Work out the finished part from the listing and answer in its coordinate system (mm). Round coordinates to 2 decimals unless told otherwise and drop trailing zeros. Order: outer loops, then holes, each group sorted by start corner. A loop starts at its lowest first (then second) coordinate and runs counter-clockwise, first axis right, second up. Notation, with made-up numbers: (19.5, 61) - (53.5, 61) arc R26 cw to (53.5, 100) - close; hole circle Ø1 at (-36.75, 45.25). An arc over 180 degrees is marked (long way). Use CSV: the item, a comma, the result in double quotes.
from build123d import *

# Parameters (mm, degrees)
SKETCH_2_R          = 38.5
SKETCH_2_R_2        = 6.5
SKETCH_2_R_3        = 1.5
EXTRUDE_1_DEPTH     = 2
CHAMFER_1_SIZE      = 2
CHAMFER_1_SIZE_2    = 1.93137755
SKETCH_3_R          = 1.7
EXTRUDE_2_DEPTH     = 2
FILLET_1_R          = 5
CUT_EXTRUDE_1_DEPTH = 10
FILLET_2_R          = 2
CUT_EXTRUDE_4_DEPTH = 10


with BuildPart() as part:
    # 草图2 → 凸台-拉伸1 (new body)
    with BuildSketch(Plane(origin=(0, 0, 0), x_dir=(1, 0, 0), z_dir=(0, 1, 0))):
        with Locations(Location((0, 0, 0), (0, 0, 270))):
            Circle(SKETCH_2_R)
        with Locations(Location((0, 0, 0), (0, 0, 270))):
            Circle(SKETCH_2_R_2, mode=Mode.SUBTRACT)
        with Locations(Location((9.5, 0, 0), (0, 0, 270))):
            Circle(SKETCH_2_R_3, mode=Mode.SUBTRACT)
        with Locations(Location((-4.75, -8.227241336, 0), (0, 0, 270))):
            Circle(SKETCH_2_R_3, mode=Mode.SUBTRACT)
        with Locations(Location((-4.75, 8.227241336, 0), (0, 0, 270))):
            Circle(SKETCH_2_R_3, mode=Mode.SUBTRACT)
    extrude(amount=EXTRUDE_1_DEPTH)

    # 倒角1
    # the kernel refuses this chamfer: 2, 1.93137755 mm, written as the material it takes off along each edge
    with BuildSketch(Plane(origin=(-4.75, 0, 8.227241336), x_dir=(0, 0, 1), z_dir=(-1, 0, 0))) as chamfer_1_piece_1:
        Polygon((1.5, CHAMFER_1_SIZE), (1.5 + CHAMFER_1_SIZE_2, 0), (1.5, 0), align=None)
    revolve(axis=Axis((-4.75, 0, 8.227241336), (0, 1, 0)), mode=Mode.SUBTRACT)
    with BuildSketch(Plane(origin=(-4.75, 0, -8.227241336), x_dir=(0, 0, 1), z_dir=(-1, 0, 0))) as chamfer_1_piece_2:
        Polygon((1.5, CHAMFER_1_SIZE), (1.5 + CHAMFER_1_SIZE_2, 0), (1.5, 0), align=None)
    revolve(axis=Axis((-4.75, 0, -8.227241336), (0, 1, 0)), mode=Mode.SUBTRACT)
    with BuildSketch(Plane(origin=(9.5, 0, 0), x_dir=(0, 0, 1), z_dir=(-1, 0, 0))) as chamfer_1_piece_3:
        Polygon((1.5, CHAMFER_1_SIZE), (1.5 + CHAMFER_1_SIZE_2, 0), (1.5, 0), align=None)
    revolve(axis=Axis((9.5, 0, 0), (0, 1, 0)), mode=Mode.SUBTRACT)

    # 草图3 → 凸台-拉伸2 (add)
    # profile 1 of 4: a face of its own
    with BuildSketch(Plane(origin=(0, 0, 0), x_dir=(1, 0, 0), z_dir=(0, 1, 0))):
        with BuildLine():
            Line((44.5, 3.5), (38.340579025, 3.5))
            ThreePointArc((38.340579025, 3.5), (38.5, 0), (38.340579025, -3.5))
            Line((38.340579025, -3.5), (44.5, -3.5))
            ThreePointArc((44.5, -3.5), (48, 0), (44.5, 3.5))
        make_face()
        with Locations(Location((44.5, 0, 0), (0, 0, 270))):
            Circle(SKETCH_3_R, mode=Mode.SUBTRACT)
    # profile 2 of 4: a face of its own
    with BuildSketch(Plane(origin=(0, 0, 0), x_dir=(1, 0, 0), z_dir=(0, 1, 0))):
        with BuildLine():
            Line((-3.5, 44.5), (-3.5, 38.340579025))
            ThreePointArc((-3.5, 38.340579025), (0, 38.5), (3.5, 38.340579025))
            Line((3.5, 38.340579025), (3.5, 44.5))
            ThreePointArc((3.5, 44.5), (0, 48), (-3.5, 44.5))
        make_face()
        with Locations(Location((0, 44.5, 0), (0, 0, 270))):
            Circle(SKETCH_3_R, mode=Mode.SUBTRACT)
    # profile 3 of 4: a face of its own
    with BuildSketch(Plane(origin=(0, 0, 0), x_dir=(1, 0, 0), z_dir=(0, 1, 0))):
        with BuildLine():
            Line((3.5, -44.5), (3.5, -38.340579025))
            ThreePointArc((3.5, -38.340579025), (0, -38.5), (-3.5, -38.340579025))
            Line((-3.5, -38.340579025), (-3.5, -44.5))
            ThreePointArc((-3.5, -44.5), (0, -48), (3.5, -44.5))
        make_face()
        with Locations(Location((0, -44.5, 0), (0, 0, 270))):
            Circle(SKETCH_3_R, mode=Mode.SUBTRACT)
    # profile 4 of 4: a face of its own
    with BuildSketch(Plane(origin=(0, 0, 0), x_dir=(1, 0, 0), z_dir=(0, 1, 0))):
        with BuildLine():
            Line((-44.5, -3.5), (-38.340579025, -3.5))
            ThreePointArc((-38.340579025, -3.5), (-38.5, 0), (-38.340579025, 3.5))
            Line((-38.340579025, 3.5), (-44.5, 3.5))
            ThreePointArc((-44.5, 3.5), (-48, 0), (-44.5, -3.5))
        make_face()
        with Locations(Location((-44.5, 0, 0), (0, 0, 270))):
            Circle(SKETCH_3_R, mode=Mode.SUBTRACT)
    extrude(amount=EXTRUDE_2_DEPTH)

    # 圆角1
    fillet_1_edges = [part.edges().sort_by_distance(p)[0] for p in [
        (38.340579025, 1, -3.5),
        (38.340579025, 1, 3.5),
        (-3.5, 1, -38.340579025),
        (3.5, 1, -38.340579025),
        (3.5, 1, 38.340579025),
        (-3.5, 1, 38.340579025),
        (-38.340579025, 1, 3.5),
        (-38.340579025, 1, -3.5),
    ]]
    fillet(fillet_1_edges, radius=FILLET_1_R)

    # 草图4 → 切除-拉伸1 (cut)
    with BuildSketch(Plane(origin=(0, 2, 0), x_dir=(1, 0, 0), z_dir=(0, 1, 0))):
        with BuildLine():
            Line((-12, 27.49545417), (-12, 12))
            Line((-12, 12), (-27.49545417, 12))
            ThreePointArc((-27.49545417, 12), (-21.213203436, 21.213203436), (-12, 27.49545417))
        make_face()
        with BuildLine():
            Line((-27.49545417, -12), (-12, -12))
            Line((-12, -12), (-12, -27.49545417))
            ThreePointArc((-12, -27.49545417), (-21.213203436, -21.213203436), (-27.49545417, -12))
        make_face()
        with BuildLine():
            Line((12, 27.49545417), (12, 12))
            Line((12, 12), (27.49545417, 12))
            ThreePointArc((27.49545417, 12), (21.213203436, 21.213203436), (12, 27.49545417))
        make_face()
        with BuildLine():
            Line((12, -12), (12, -27.49545417))
            ThreePointArc((12, -27.49545417), (21.213203436, -21.213203436), (27.49545417, -12))
            Line((27.49545417, -12), (12, -12))
        make_face()
    extrude(amount=-CUT_EXTRUDE_1_DEPTH, mode=Mode.SUBTRACT)

    # 圆角2
    fillet_2_edges = [part.edges().sort_by_distance(p)[0] for p in [
        (-12, 1, 27.49545417),
        (-27.49545417, 1, 12),
        (-12, 1, 12),
        (12, 1, -27.49545417),
        (27.49545417, 1, -12),
        (12, 1, -12),
        (27.49545417, 1, 12),
        (12, 1, 27.49545417),
        (12, 1, 12),
        (-27.49545417, 1, -12),
        (-12, 1, -27.49545417),
        (-12, 1, -12),
    ]]
    fillet(fillet_2_edges, radius=FILLET_2_R)

    # 草图5 → 切除-拉伸4 (cut)
    with BuildSketch(Plane(origin=(0, 2, 0), x_dir=(1, 0, 0), z_dir=(0, 1, 0))):
        with BuildLine():
            Line((3, 32), (3, 20))
            ThreePointArc((3, 20), (0, 17), (-3, 20))
            Line((-3, 20), (-3, 32))
            ThreePointArc((-3, 32), (0, 35), (3, 32))
        make_face()
        with BuildLine():
            Line((32, 3), (20, 3))
            ThreePointArc((20, 3), (17, 0), (20, -3))
            Line((20, -3), (32, -3))
            ThreePointArc((32, -3), (35, 0), (32, 3))
        make_face()
        with BuildLine():
            Line((-3, -32), (-3, -20))
            ThreePointArc((-3, -20), (0, -17), (3, -20))
            Line((3, -20), (3, -32))
            ThreePointArc((3, -32), (0, -35), (-3, -32))
        make_face()
        with BuildLine():
            Line((-32, -3), (-20, -3))
            ThreePointArc((-20, -3), (-17, 0), (-20, 3))
            Line((-20, 3), (-32, 3))
            ThreePointArc((-32, 3), (-35, 0), (-32, -3))
        make_face()
    extrude(amount=-CUT_EXTRUDE_4_DEPTH, mode=Mode.SUBTRACT)


solid = part.part
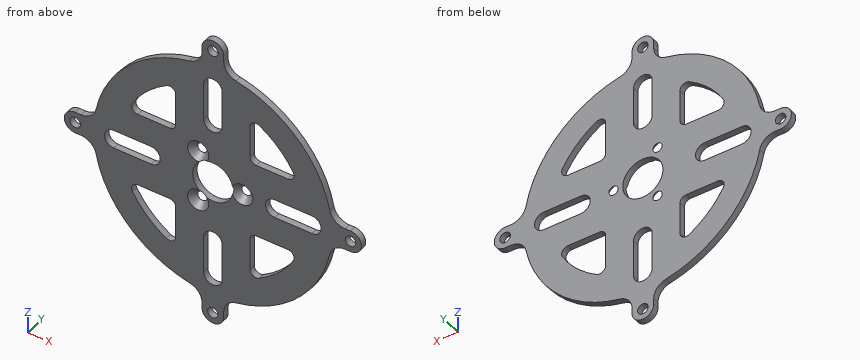
(1) Find the intervals of material crossed by L1, parallel to X at y = 0.45, z = -23.5; L2, parallel to Z at x = -6, y = 0.55; L3, parallel to X at y = 1.4, z = 44.5, in increasing order. Write a range as from..to.
Findings below:
L1,"x = -30.5..-18.65, -12..-3, 3..12, 18.65..30.5"
L2,"z = -38.33..-10.84, -5.61..-2.5, 2.5..5.61, 10.84..38.33"
L3,"x = -3.5..-1.7, 1.7..3.5"
(2) Each of these flat-tipped pins is pushed along its axis until it touches: pin 1 (0.9 mm diameter, centred on x = -44, y = 1.5, fed in from +Z); pin 2 (4 mm diameter, centred on x = -21.5, z = 17, fed in from +Y); pin 3 (0.6 mm diameter, centred on y = 0.5, z = -43.5, fed in from +X); pin 4 (0.6 mm diameter, centred on y = 1, z = -21.5, fed in from -X). Where does it stop, or does it pass through?
Findings below:
pin 1,"stops at z = 3.5"
pin 2,"passes through"
pin 3,"stops at x = 3.5"
pin 4,"stops at x = -32.14"
(3) Find section C-C (y = 0.35). State how many separate pieces and enclosed holes the cut face has, and give its area (3 significant figures).
Findings below:
separate pieces,"1"
enclosed holes,"13"
area,"3,690 mm²"
(4) Find section A-A (z = 0). Determine the outline of the cut face in (x, y), and give its area (3 significant figures).
Findings below:
outline,"(-48, 0) - (-46.2, 0) - (-46.2, 2) - (-48, 2) - close; (-42.8, 0) - (-35, 0) - (-35, 2) - (-42.8, 2) - close; (-17, 0) - (-6.5, 0) - (-6.5, 2) - (-17, 2) - close; (6.5, 0.45) - (8, 2) - (6.5, 2) - close; (11, 2) - (12.93, 0) - (17, 0) - (17, 2) - close; (35, 0) - (42.8, 0) - (42.8, 2) - (35, 2) - close; (46.2, 0) - (48, 0) - (48, 2) - (46.2, 2) - close"
area,"70.6 mm²"
(5) Find section B-B (z = 29). Determine the outline of the cut face in (x, y), and give its area (3 significant figures).
Findings below:
outline,"(-25.32, 0) - (-3, 0) - (-3, 2) - (-25.32, 2) - close; (3, 0) - (25.32, 0) - (25.32, 2) - (3, 2) - close"
area,"89.3 mm²"
(6) Find section D-D (z = -36.5). Determine the outline of the cut face in (x, y).
Findings below:
outline,"(-12.25, 0) - (12.25, 0) - (12.25, 2) - (-12.25, 2) - close"
